```python
from build123d import *

# Parameters (mm, degrees)
SKETCH2_R                = 2
BOSS_EXTRUDE1_DEPTH      = 30
SKETCH3_W                = 7
SKETCH3_H                = 12
SKETCH3_W_2              = 8
CUT_EXTRUDE1_DEPTH       = 60
CUT_EXTRUDE2_DEPTH       = 42
CUT_EXTRUDE5_DEPTH       = 70
CUT_EXTRUDE9_DEPTH       = 70
CUT_EXTRUDE10_DEPTH      = 7
CUT_EXTRUDE11_DEPTH      = 17
CUT_EXTRUDE11_DEPTH_BACK = 17
SKETCH9_W                = 8
SKETCH9_H                = 2


with BuildPart() as part:
    # Sketch2 → Boss-Extrude1 (new body)
    with BuildSketch(Plane.YZ):
        with BuildLine():
            Line((0, -4), (-78, -4))
            ThreePointArc((-78, -4), (-80.828427125, -2.828427125), (-82, 0))
            Line((-82, 0), (-78.449171497, 15.448029549))
            ThreePointArc((-78.449171497, 15.448029549), (-77.745781061, 16.56461802), (-76.5, 17))
            Line((-76.5, 17), (-5.35, 33.4))
            ThreePointArc((-5.35, 33.4), (-2.521572875, 32.228427125), (-1.35, 29.4))
            Line((-1.35, 29.4), (4, 0))
            ThreePointArc((4, 0), (2.828427125, -2.828427125), (0, -4))
        make_face()
        with Locations(Location((0, 0, 0), (0, 0, 270))):
            Circle(SKETCH2_R, mode=Mode.SUBTRACT)
        with Locations(Location((-78, 0, 0), (0, 0, 270))):
            Circle(SKETCH2_R, mode=Mode.SUBTRACT)
    extrude(amount=BOSS_EXTRUDE1_DEPTH)

    # Sketch3 → Cut-Extrude1 (cut)
    with BuildSketch(Plane(origin=(0, 0, 46), x_dir=(-1, 0, 0), z_dir=(0, 0, -1))):
        Polygon((0, 0), (0, 4), (-7, 4), (-7, -8), (0, -8), align=None)
        with Locations((-26.5, -2)):
            Rectangle(SKETCH3_W, SKETCH3_H)
        with Locations((-15, -2)):
            Rectangle(SKETCH3_W_2, SKETCH3_H)
    extrude(amount=CUT_EXTRUDE1_DEPTH, mode=Mode.SUBTRACT)

    # Sketch4 → Cut-Extrude2 (cut)
    with BuildSketch(Plane(origin=(0, 0, 46), x_dir=(-1, 0, 0), z_dir=(0, 0, -1))):
        Polygon((-15, 3.93673286), (-4, 3.93673286), (-4, -82.06326714), (-25.011555161, -82.06326714), (-26, 3.93673286), align=None)
    extrude(amount=CUT_EXTRUDE2_DEPTH, mode=Mode.SUBTRACT)

    # Sketch6 → Cut-Extrude5 (cut)
    with BuildSketch(Plane(origin=(0, 0, 46), x_dir=(-1, 0, 0), z_dir=(0, 0, -1))):
        Polygon((-15, -62), (-4, -62), (-4, -102), (-26, -102), (-26, -62), align=None)
    extrude(amount=CUT_EXTRUDE5_DEPTH, mode=Mode.SUBTRACT)

    # Sketch7 → Cut-Extrude9 (cut)
    with BuildSketch(Plane(origin=(0, 0, 0), x_dir=(0, -1, 0), z_dir=(-1, 0, 0))):
        with BuildLine():
            Line((8, 28.29), (8, 32.789177793))
            Line((8, 32.789177793), (76.5, 17))
            ThreePointArc((76.5, 17), (77.745781061, 16.56461802), (78.449171497, 15.448029549))
            Line((78.449171497, 15.448029549), (79.020603501, 12.961990453))
            Line((79.020603501, 12.961990453), (8, 28.29))
        make_face()
    extrude(amount=-CUT_EXTRUDE9_DEPTH, mode=Mode.SUBTRACT)

    # Sketch8 → Cut-Extrude10 (cut)
    with BuildSketch(Plane(origin=(0, 0, 0), x_dir=(0, -1, 0), z_dir=(-1, 0, 0))):
        with BuildLine():
            Line((8, 28.29), (25.445762173, 24.608385924))
            ThreePointArc((25.445762173, 24.608385924), (8.078114511, 11.960989597), (22.46, -4))
            Line((22.46, -4), (-8.040982842, -4))
            Line((-8.040982842, -4), (-8.040982842, 32.936104238))
            Line((-8.040982842, 32.936104238), (8, 28.29))
        make_face()
    cut_extrude10 = extrude(amount=-CUT_EXTRUDE10_DEPTH, mode=Mode.SUBTRACT)

    # Mirror1: Cut-Extrude10 across plane
    add(cut_extrude10.mirror(Plane(origin=(15, 0, 0), x_dir=(0, 0, 1), z_dir=(1, 0, 0))), mode=Mode.SUBTRACT)

    # Sketch9 → Cut-Extrude11 (cut, two sides: drawn at the far end of the back side and taken through both)
    with BuildSketch(Plane(origin=(0, 0, 0), x_dir=(0, 1, 0), z_dir=(0, 0, 1)).offset(-CUT_EXTRUDE11_DEPTH_BACK)):
        with Locations((-78, -1)):
            Rectangle(SKETCH9_W, SKETCH9_H)
        with Locations((-78, -29)):
            Rectangle(SKETCH9_W, SKETCH9_H)
    extrude(amount=CUT_EXTRUDE11_DEPTH + CUT_EXTRUDE11_DEPTH_BACK, mode=Mode.SUBTRACT)


solid = part.part
```
Input: part model. Units: mm. Frame: model coordinates. A direction names the side the tool comes from. Give positions to 0.01 mm unless a question says otherwise; leave off trailing zeros. Order: outer loops, then holes, each group sorted by start corner. A loop starts at its lowest first (then second) coordinate and runs counter-clockwise, first axis right, second up. Notation, with made-up numbers: M -29,-8 L 19,-8 A7 ccw 19,-4 Z; hole C 49.5,-12 d2. An arc over 180 degrees is marked long. One line per question, with ' | ' between items.
1) Section D-D on y = -48. Output: boundary loops of the cut face in (x, z).
Filled in:
outline: M 0,-4 L 30,-4 L 30,19.66 L 25.4,19.66 L 25.4,4 L 4,4 L 4,19.66 L 0,19.66 Z
2) Section C-C on x = 17. Output: boundary loops of the cut face in (y, z).
Filled in:
outline: M -62,-4 L -8,-4 L -8,4 L -62,4 Z
3) Contact query for flat-ended pins moving along their axis: P1, Ø10, axis at x = 6.5, y = -36, coming from the +Z side; P2, Ø4.5, axis at y = -78, z = 0, coming from the +X side; P3, Ø3.5, axis at y = 0, z = 0, coming from the -X side; P4, Ø2, axis at x = 1.5, z = 4, coming from the -Y side. Output: stop coordinate, or through.
Filled in:
P1: stops at z = 23.18 | P2: stops at x = 28 | P3: passes through | P4: stops at y = -81.28
4) Section A-A on y = -68. Output: boundary loops of the cut face in (x, z).
Filled in:
outline: M 0,-4 L 4,-4 L 4,15.34 L 0,15.34 Z; M 26,-4 L 30,-4 L 30,15.34 L 26,15.34 Z
5) Access query for faces 4 (the face through (26, -70, 6)), 5 (the face through (28, -77, 5)), 6 (the face through (11, -3, 0)), 7 (the face through (23, -6, 0)). Directions: +Z, -Z, +X, -X, +Y, -Y. A direction counts if a zero-diameter tool reaches every point of the face in a straight line with its end or side. Return the directions, or none.
Filled in:
face 4: +Z, -Z, -Y | face 5: +Z, -Z, +X, -Y | face 6: +Z, -Z, +Y | face 7: -Z, +X, +Y
6) Draft query along Z for faces 1 (the face through (27.588, -51.891, 18.817)), 2 (the face through (21, -2, 0)), 3 (the face through (29, -74, 5)). Return one class per face: pulls with the +Z half, pulls with the -Z half, needs draft (parallel to the pull), parting line crosses it, or undercut.
Filled in:
face 1: pulls with the +Z half | face 2: undercut | face 3: needs draft
7) Ray query, L1, parallel to Y at x = 21.75, z = 0; L2, parallel to X at y = -72, z = 6.5; L3, parallel to Z at x = 21.95, y = 0. Return the intervals inside material, ascending.
Filled in:
L1: y = -62 to -2, 2 to 4 | L2: x = 0 to 4, 26 to 30 | L3: z = -4 to -2, 2 to 4
8) Section B-B on z = 21. Output: boundary loops of the cut face in (x, y).
Filled in:
outline: M 0,-41.78 L 4,-41.78 L 4,-12.56 L 0,-12.56 Z; M 25.47,-41.78 L 30,-41.78 L 30,-12.56 L 25.81,-12.56 Z
